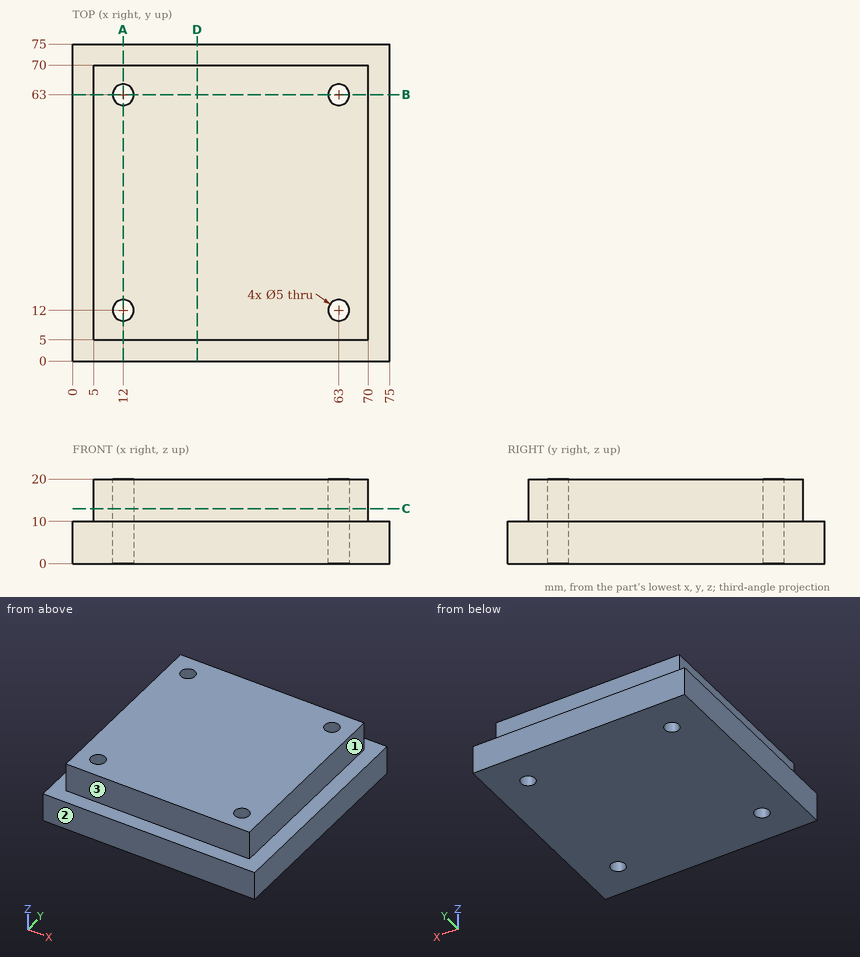
Study the drawing (mm; zero at the part's minimum x, y, z) and answer. A direction names the side the tool comes from. Give positions to 0.01 mm unless a question says otherwise; leave off trailing zeros. Write each loop counter-clockwise with the first axis right and the second up, starting at its lowest first coordinate (ties: lowest second). Pieces come first, ordered by that corner, then holes.
(1) The part is cut by section A-A on x = 12. Write down the section's boundary in (y, z), plus the area to 3 significant figures.
Final values:
outline: (0, 0) - (9.5, 0) - (9.5, 20) - (5, 20) - (5, 10) - (0, 10) - close; (14.5, 0) - (60.5, 0) - (60.5, 20) - (14.5, 20) - close; (65.5, 0) - (75, 0) - (75, 10) - (70, 10) - (70, 20) - (65.5, 20) - close
area: 1,200 mm2
(2) Flat-ended cylindrical pins translate along their axes: pin 1 Ø8 at (y, z) = (53.5, 13) entering from -X; pin 2 Ø8 at (x, z) = (49.5, 15) entering from +Y; pin 3 Ø8 at (y, z) = (13, 15) entering from -X; pin 4 Ø5 at (x, z) = (41, 14) entering from -Y. Find the tip coordinate at first contact, or state that the pin passes through.
Final values:
pin 1: stops at x = 0
pin 2: stops at y = 70
pin 3: stops at x = 5
pin 4: stops at y = 5
(3) The part is cut by section C-C on z = 13. Write down the section's boundary in (x, y), plus the area to 3 significant figures.
Final values:
outline: (5, 5) - (70, 5) - (70, 70) - (5, 70) - close; hole circle Ø5 at (12, 12); hole circle Ø5 at (12, 63); hole circle Ø5 at (63, 12); hole circle Ø5 at (63, 63)
area: 4,150 mm2
(4) Which of the six approach directions +Z, -Z, +X, -X, +Y, -Y give full straight-line access (tool end or side, diameter ignored) to the marked faces 1, 2 and 3?
Final values:
face 1: +Z, +X, +Y, -Y
face 2: +Z, -Z, +X, -X, -Y
face 3: +Z, +X, -X, -Y
(5) Straight lines are drawn through the part: line 1 (Y direction, x = 63, z = 15.75); line 2 (Y direction, x = 63, z = 9.25); line 3 (Y direction, x = 35, z = 11). For each, find the intervals that lie inside material, in ascending order.
Final values:
line 1: y = 5 to 9.5, 14.5 to 60.5, 65.5 to 70
line 2: y = 0 to 9.5, 14.5 to 60.5, 65.5 to 75
line 3: y = 5 to 70
(6) The part is cut by section D-D on x = 29.5. Write down the section's boundary in (y, z).
Final values:
outline: (0, 0) - (75, 0) - (75, 10) - (70, 10) - (70, 20) - (5, 20) - (5, 10) - (0, 10) - close
